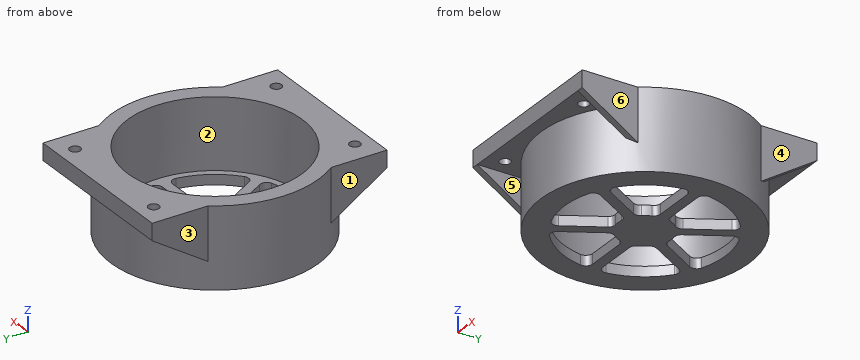
```python
from build123d import *

# Parameters (mm, degrees)
BOSS_EXTRUDE1_DEPTH     = 5
RIB4_REACH              = 72.264
SKETCH3_WALL_W          = 162.412301062
SKETCH3_WALL_H          = 2
MIRROR2_COPY_1_REACH    = 72.264
MIRROR2_COPY_1_SKETCH_W = 162.412301062
MIRROR2_COPY_1_SKETCH_H = 2
CUT_EXTRUDE1_DEPTH      = 52.254268115
SKETCH5_R               = 1.6
CUT_EXTRUDE2_DEPTH      = 53.554733374


with BuildPart() as part:
    # Sketch1 → Revolve1 (revolve)
    with BuildSketch(Plane(origin=(0, 0, 0), x_dir=(0, 0, -1), z_dir=(1, 0, 0)), mode=Mode.PRIVATE) as revolve1_sk:
        Polygon((0, 0), (0, 31), (-24, 31), (-24, 26), (-3, 26), (-3, 0), align=None)
    revolve(revolve1_sk.sketch.rotate(Axis((0, 0, 0), (0, 0, 1)), 90), axis=Axis((0, 0, 0), (0, 0, 1)))

    # Sketch2 → Boss-Extrude1 (add)
    with BuildSketch(Plane.XY.offset(24)):
        with BuildLine():
            Line((25, 35), (-25, 35))
            Line((-25, 35), (-25, 18.33030278))
            ThreePointArc((-25, 18.33030278), (0, 31), (25, 18.33030278))
            Line((25, 18.33030278), (25, 35))
        make_face()
        with BuildLine():
            Line((25, -35), (25, -18.33030278))
            ThreePointArc((25, -18.33030278), (0, -31), (-25, -18.33030278))
            Line((-25, -18.33030278), (-25, -35))
            Line((-25, -35), (25, -35))
        make_face()
    extrude(amount=-BOSS_EXTRUDE1_DEPTH)

    # Sketch3 wall → Rib4 (add, up to next)
    with BuildSketch(Plane(origin=(25, 26.66515139, 13.579588783), x_dir=(0, -0.838316763898, -0.54518345845), z_dir=(0, 0.54518345845, -0.838316763898)), mode=Mode.PRIVATE) as rib4_sk1:
        with Locations((0, 1)):
            Rectangle(SKETCH3_WALL_W, SKETCH3_WALL_H)
    rib4_tool1 = extrude(rib4_sk1.sketch, amount=-RIB4_REACH, mode=Mode.PRIVATE) - part.part
    rib4 = rib4_tool1.solids().sort_by_distance((25, 26.66515139, 13.579588783))[0]
    add(rib4)

    # Mirror1: Rib4 across plane
    add(rib4.mirror(Plane.ZX))

    # Mirror2: Rib4 across plane
    add(rib4.mirror(Plane(origin=(0, 0, 0), x_dir=(0, 0, 1), z_dir=(1, 0, 0))))

    # Mirror2 copy 1 sketch → Mirror2 copy 1 (add, up to next)
    with BuildSketch(Plane(origin=(-25, -26.66515139, 13.579588783), x_dir=(0, 0.838316763898, -0.54518345845), z_dir=(0, -0.54518345845, -0.838316763898)), mode=Mode.PRIVATE) as mirror2_copy_1_sk1:
        with Locations((0, 1)):
            Rectangle(MIRROR2_COPY_1_SKETCH_W, MIRROR2_COPY_1_SKETCH_H)
    mirror2_copy_1_tool1 = extrude(mirror2_copy_1_sk1.sketch, amount=-MIRROR2_COPY_1_REACH, mode=Mode.PRIVATE) - part.part
    add(mirror2_copy_1_tool1.solids().sort_by_distance((-25, -26.66515139, 13.579588783))[0])

    # Sketch4 → Cut-Extrude1 (cut, through all)
    with BuildSketch(Plane.XY.offset(3)):
        with BuildLine():
            Line((-9.560865209, 19.559904306), (-3.384710393, 8.86249037))
            ThreePointArc((-3.384710393, 8.86249037), (-2.50559682, 8.053485651), (-1.322127668, 7.889992296))
            ThreePointArc((-1.322127668, 7.889992296), (0, 8), (1.322127668, 7.889992296))
            ThreePointArc((1.322127668, 7.889992296), (2.50559682, 8.053485651), (3.384710393, 8.86249037))
            Line((3.384710393, 8.86249037), (9.560865209, 19.559904306))
            ThreePointArc((9.560865209, 19.559904306), (9.713197693, 21.230053251), (8.540524801, 22.428986516))
            ThreePointArc((8.540524801, 22.428986516), (0, 24), (-8.540524801, 22.428986516))
            ThreePointArc((-8.540524801, 22.428986516), (-9.713197693, 21.230053251), (-9.560865209, 19.559904306))
        make_face()
        with BuildLine():
            Line((21.719806629, 1.5), (9.367496998, 1.5))
            ThreePointArc((9.367496998, 1.5), (8.227321572, 1.856832327), (7.493997598, 2.8))
            ThreePointArc((7.493997598, 2.8), (6.92820323, 4), (6.17186993, 5.089992296))
            ThreePointArc((6.17186993, 5.089992296), (5.721724752, 6.196653323), (5.982786604, 7.36249037))
            Line((5.982786604, 7.36249037), (12.15894142, 18.059904306))
            ThreePointArc((12.15894142, 18.059904306), (13.529166592, 19.02690258), (15.153809703, 18.610804697))
            ThreePointArc((15.153809703, 18.610804697), (20.784609691, 12), (23.694334504, 3.818181818))
            ThreePointArc((23.694334504, 3.818181818), (23.242364286, 2.203150671), (21.719806629, 1.5))
        make_face()
        with BuildLine():
            Line((12.15894142, -18.059904306), (5.982786604, -7.36249037))
            ThreePointArc((5.982786604, -7.36249037), (5.721724752, -6.196653323), (6.17186993, -5.089992296))
            ThreePointArc((6.17186993, -5.089992296), (6.92820323, -4), (7.493997598, -2.8))
            ThreePointArc((7.493997598, -2.8), (8.227321572, -1.856832327), (9.367496998, -1.5))
            Line((9.367496998, -1.5), (21.719806629, -1.5))
            ThreePointArc((21.719806629, -1.5), (23.242364286, -2.203150671), (23.694334504, -3.818181818))
            ThreePointArc((23.694334504, -3.818181818), (20.784609691, -12), (15.153809703, -18.610804697))
            ThreePointArc((15.153809703, -18.610804697), (13.529166592, -19.02690258), (12.15894142, -18.059904306))
        make_face()
        with BuildLine():
            Line((-9.560865209, -19.559904306), (-3.384710393, -8.86249037))
            ThreePointArc((-3.384710393, -8.86249037), (-2.50559682, -8.053485651), (-1.322127668, -7.889992296))
            ThreePointArc((-1.322127668, -7.889992296), (0, -8), (1.322127668, -7.889992296))
            ThreePointArc((1.322127668, -7.889992296), (2.50559682, -8.053485651), (3.384710393, -8.86249037))
            Line((3.384710393, -8.86249037), (9.560865209, -19.559904306))
            ThreePointArc((9.560865209, -19.559904306), (9.713197693, -21.230053251), (8.540524801, -22.428986516))
            ThreePointArc((8.540524801, -22.428986516), (0, -24), (-8.540524801, -22.428986516))
            ThreePointArc((-8.540524801, -22.428986516), (-9.713197693, -21.230053251), (-9.560865209, -19.559904306))
        make_face()
        with BuildLine():
            Line((-21.719806629, -1.5), (-9.367496998, -1.5))
            ThreePointArc((-9.367496998, -1.5), (-8.227321572, -1.856832327), (-7.493997598, -2.8))
            ThreePointArc((-7.493997598, -2.8), (-6.92820323, -4), (-6.17186993, -5.089992296))
            ThreePointArc((-6.17186993, -5.089992296), (-5.721724752, -6.196653323), (-5.982786604, -7.36249037))
            Line((-5.982786604, -7.36249037), (-12.15894142, -18.059904306))
            ThreePointArc((-12.15894142, -18.059904306), (-13.529166592, -19.02690258), (-15.153809703, -18.610804697))
            ThreePointArc((-15.153809703, -18.610804697), (-20.784609691, -12), (-23.694334504, -3.818181818))
            ThreePointArc((-23.694334504, -3.818181818), (-23.242364286, -2.203150671), (-21.719806629, -1.5))
        make_face()
        with BuildLine():
            Line((-12.15894142, 18.059904306), (-5.982786604, 7.36249037))
            ThreePointArc((-5.982786604, 7.36249037), (-5.721724752, 6.196653323), (-6.17186993, 5.089992296))
            ThreePointArc((-6.17186993, 5.089992296), (-6.92820323, 4), (-7.493997598, 2.8))
            ThreePointArc((-7.493997598, 2.8), (-8.227321572, 1.856832327), (-9.367496998, 1.5))
            Line((-9.367496998, 1.5), (-21.719806629, 1.5))
            ThreePointArc((-21.719806629, 1.5), (-23.242364286, 2.203150671), (-23.694334504, 3.818181818))
            ThreePointArc((-23.694334504, 3.818181818), (-20.784609691, 12), (-15.153809703, 18.610804697))
            ThreePointArc((-15.153809703, 18.610804697), (-13.529166592, 19.02690258), (-12.15894142, 18.059904306))
        make_face()
    extrude(amount=-CUT_EXTRUDE1_DEPTH, mode=Mode.SUBTRACT)

    # Sketch5 → Cut-Extrude2 (cut, through all)
    with BuildSketch(Plane.XY.offset(24)):
        with Locations((-18, 30)):
            Circle(SKETCH5_R)
        with Locations((18, 30)):
            Circle(SKETCH5_R)
        with Locations((18, -30)):
            Circle(SKETCH5_R)
        with Locations((-18, -30)):
            Circle(SKETCH5_R)
    extrude(amount=-CUT_EXTRUDE2_DEPTH, mode=Mode.SUBTRACT)


solid = part.part
```
The model under review builds one solid part; all positions refer to its coordinate system, in mm. Face numbers are marked on the shaded views. A direction names the side the tool comes from. Coordinates: 2 decimals unless noted, no trailing zeros. Write each loop counter-clockwise with the first axis right and the second up, starting at its lowest first coordinate (ties: lowest second). Pieces come first, ordered by that corner, then holes. Notation, with made-up numbers: (23.5, 51) - (45.5, 51) arc R20 ccw to (45.5, 58) - close; hole circle Ø8 at (26, 39.5). An arc over 180 degrees is marked (long way). Answer in a Markdown table with one row per item. Add a question column.
Q1. For the marked faces 3, 4, 5 and 6, list the 3-axis set-ups (+Z, -Z, +X, -X, +Y, -Y) from which the entire face can be reached by the end or side of a thin tool; tool diameter is ignored.
Q2. To check wall thickness, follow line 1 along Y through (x, z) = (0, 9.5); line 2 along Y through (x, z) = (18, 22.65); line 3 along X through (y, z) = (-5, 21). State the ranges of each line that lie inside material, in increasing order. Write a range as from..to.
Q3. Consider section D-D on y = 0. Give the boundary of the cut face in (x, z).
Q4. Consider section C-C on y = -12. Give the boundary of the cut face in (x, z).
Q5. Consider section A-A on x = 0. Give the boundary of the cut face in (y, z), then the cut area to 3 significant figures.
Q6. Consider section B-B on x = 18. Give the boundary of the cut face in (y, z), then the cut area to 3 significant figures.
Q7. Clearance check with flat-ended pins moving along their axes: pin 1 (8 mm diameter, centred on y = -30, z = 16.5, fed in from +X); pin 2 (3.5 mm diameter, centred on x = -14.5, z = 1, fed in from -Y); pin 3 (12 mm diameter, centred on x = 15.5, z = 7.5, fed in from +Y). State where each tip first meets the part, or that it passes through.
Q8. Draft analysis for pull direction Y (two halves, no side actions). For the marked faces 1 and 2, state which applies: +Y half, -Y half, draft (parallel to the pull), parting line (faces both ways), or undercut.
Answers below:
| question | item | result |
|---|---|---|
| 1 | face 3 | +Z, -Z, -X, +Y |
| 1 | face 4 | +Z, -Z, +X, +Y |
| 1 | face 5 | -Z, -Y |
| 1 | face 6 | +Z, -Z, +X, -Y |
| 2 | line 1 | -31..-26, 26..31 |
| 2 | line 2 | -35..-31.6, -28.4..-18.76, 18.76..28.4, 31.6..35 |
| 2 | line 3 | -30.59..-25.51, 25.51..30.59 |
| 3 | outline | (-31, 0) - (31, 0) - (31, 24) - (26, 24) - (26, 3) - (-26, 3) - (-26, 24) - (-31, 24) - close |
| 4 | outline | (-28.58, 0) - (-20.78, 0) - (-20.78, 3) - (-23.07, 3) - (-23.07, 24) - (-28.58, 24) - close; (-8.66, 0) - (-5.2, 0) - (-5.2, 3) - (-8.66, 3) - close; (5.2, 0) - (8.66, 0) - (8.66, 3) - (5.2, 3) - close; (20.78, 0) - (28.58, 0) - (28.58, 24) - (23.07, 24) - (23.07, 3) - (20.78, 3) - close |
| 5 | outline | (-35, 19) - (-31, 19) - (-31, 0) - (-24, 0) - (-24, 3) - (-26, 3) - (-26, 24) - (-35, 24) - close; (-8, 0) - (8, 0) - (8, 3) - (-8, 3) - close; (24, 0) - (31, 0) - (31, 19) - (35, 19) - (35, 24) - (26, 24) - (26, 3) - (24, 3) - close |
| 5 | area | 340 mm² |
| 6 | outline | (-35, 19) - (-31.6, 19) - (-31.6, 24) - (-35, 24) - close; (-28.4, 19) - (-25.24, 19) - (-25.24, 0) - (-15.87, 0) - (-15.87, 3) - (-18.76, 3) - (-18.76, 24) - (-28.4, 24) - close; (-1.5, 0) - (1.5, 0) - (1.5, 3) - (-1.5, 3) - close; (15.87, 0) - (25.24, 0) - (25.24, 19) - (28.4, 19) - (28.4, 24) - (18.76, 24) - (18.76, 3) - (15.87, 3) - close; (31.6, 19) - (35, 19) - (35, 24) - (31.6, 24) - close |
| 6 | area | 403 mm² |
| 7 | pin 1 | x = 25 |
| 7 | pin 2 | y = -28.26 |
| 7 | pin 3 | y = 29.51 |
| 8 | face 1 | draft |
| 8 | face 2 | undercut |
